```python
from build123d import *

# Parameters (mm, degrees)
EXTRUDE_START   = -16
SKETCH_1_R      = 1.75
SKETCH_1_R_2    = 4.025
EXTRUDE_1_DEPTH = 3


with BuildPart() as part:
    # ｽｹｯﾁ1 → ﾎﾞｽ - 押し出し1 (new body)
    with BuildSketch(Plane.XY.offset(EXTRUDE_START)):
        Polygon((8.636200269, 92.596668368), (0, 38), (0, 21.596668368), (68.636200269, 21.596668368), (73.636200269, 21.596668368), (73.636200269, 97.596668368), (60, 97.596668368), (46.2, 97.596668368), (46.2, 92.596668368), (46.2, 58.596668368), (31.2, 58.596668368), (31.2, 92.596668368), (31.2, 97.596668368), (8.636200269, 97.596668368), align=None)
        with Locations((14.636200269, 86.596668368)):
            Circle(SKETCH_1_R, mode=Mode.SUBTRACT)
        with Locations((14.636200269, 68.596668368)):
            Circle(SKETCH_1_R, mode=Mode.SUBTRACT)
        with Locations((8, 30)):
            Circle(SKETCH_1_R_2, mode=Mode.SUBTRACT)
        with Locations((71.136200269, 26.596668368)):
            Circle(SKETCH_1_R, mode=Mode.SUBTRACT)
        with Locations((71.136200269, 87.596668368)):
            Circle(SKETCH_1_R, mode=Mode.SUBTRACT)
        with Locations((68.636200269, 95.096668368)):
            Circle(SKETCH_1_R, mode=Mode.SUBTRACT)
        with Locations((13.636200269, 95.202370808)):
            Circle(SKETCH_1_R, mode=Mode.SUBTRACT)
    extrude(amount=-EXTRUDE_1_DEPTH)


solid = part.part
```
Part model, mm, in its own coordinate system. A direction names the side the tool comes from. Round coordinates to 2 decimals unless told otherwise and drop trailing zeros. Loops run counter-clockwise (first coordinate to the right, second up) from the corner with the lowest first, then second, coordinate; pieces in that order, holes last. Notation, with made-up numbers: (40, 79) -> (78, 79) arc R24 cw to (78, 101) -> close; hole circle Ø11 at (47, 81). An arc over 180 degrees is marked (long way). Use a Markdown table: item, result.
1) Cut at C-C, the plane z = -17.9. List the corners of the cut face in (x, y) (3 decimals).
The answers:
| item | result |
|---|---|
| outline | (0, 21.597) -> (73.636, 21.597) -> (73.636, 97.597) -> (46.2, 97.597) -> (46.2, 58.597) -> (31.2, 58.597) -> (31.2, 97.597) -> (8.636, 97.597) -> (8.636, 92.597) -> (0, 38) -> close; hole circle Ø8.05 at (8, 30); hole circle Ø3.5 at (13.636, 95.202); hole circle Ø3.5 at (14.636, 68.597); hole circle Ø3.5 at (14.636, 86.597); hole circle Ø3.5 at (68.636, 95.097); hole circle Ø3.5 at (71.136, 26.597); hole circle Ø3.5 at (71.136, 87.597) |
2) Tool access for faces 5 (the flat face through (8.636, 95, -17)), 6 (the flat face through (39, 58.597, -17)), 7 (the flat face through (0, 30, -17)): list every direction of +Z, -Z, +X, -X, +Y, -Y with a clear straight run to the whole face (end or side of a thin tool).
The answers:
| item | result |
|---|---|
| face 5 | +Z, -Z, -X, +Y |
| face 6 | +Z, -Z, +Y |
| face 7 | +Z, -Z, -X, +Y, -Y |
3) Cut at D-D, the plane x = 38.5. List the corners of the cut face in (y, z), and give its area (3 significant figures).
The answers:
| item | result |
|---|---|
| outline | (21.6, -19) -> (58.6, -19) -> (58.6, -16) -> (21.6, -16) -> close |
| area | 111 mm2 |
4) Cut at A-A, the plane y = 30. List the corners of the cut face in (x, z) (3 decimals), and give its area (3 significant figures).
The answers:
| item | result |
|---|---|
| outline | (0, -19) -> (3.975, -19) -> (3.975, -16) -> (0, -16) -> close; (12.025, -19) -> (73.636, -19) -> (73.636, -16) -> (12.025, -16) -> close |
| area | 197 mm2 |
5) Drop flat-ended pins along their axis: pin 1 Ø6.5 at (x, y) = (8, 30) entering from -Z; pin 2 Ø0.9 at (y, z) = (86.5, -18) entering from -X; pin 3 Ø0.9 at (x, z) = (38.5, -17.5) entering from +Y; pin 4 Ø1.5 at (y, z) = (96.5, -17.5) entering from -X. Give the stop position or say it passes through.
The answers:
| item | result |
|---|---|
| pin 1 | passes through |
| pin 2 | stops at x = 7.6 |
| pin 3 | stops at y = 58.6 |
| pin 4 | stops at x = 8.64 |
6) Pull direction X, two halves, no side cores. Call faces 1 (the flat face through (4.38, 65.68, -17.48)), 2 (the flat face through (46.2, 78, -17)), 3 (the cylindrical face through (16.253, 67.926, -17.479)), 4 (the flat face through (36, 52, -16)): pulls with the +X half, pulls with the -X half, needs draft (parallel to the pull), parting line crosses it, or undercut.
The answers:
| item | result |
|---|---|
| face 1 | pulls with the -X half |
| face 2 | undercut |
| face 3 | undercut |
| face 4 | needs draft |
7) Probe line 1 (Y direction, x = 15, z = -16.3); line 2 (X direction, y = 68, z = -17.85); line 3 (X direction, y = 67, z = -18.45). List the from-to ranges inside material, lowest first. Write a range as [from, to].
The answers:
| item | result |
|---|---|
| line 1 | y = [21.6, 66.88], [70.31, 84.88], [88.31, 94.11], [96.3, 97.6] |
| line 2 | x = [4.75, 12.99], [16.28, 31.2], [46.2, 73.64] |
| line 3 | x = [4.59, 13.92], [15.35, 31.2], [46.2, 73.64] |
8) Cut at B-B, the plane x = 68. List the corners of the cut face in (y, z), and give its area (3 significant figures).
The answers:
| item | result |
|---|---|
| outline | (21.6, -19) -> (93.47, -19) -> (93.47, -16) -> (21.6, -16) -> close; (96.73, -19) -> (97.6, -19) -> (97.6, -16) -> (96.73, -16) -> close |
| area | 218 mm2 |
